Answer from the drawing. Dimensions are ordinates in mm from the lowest x, y and z of the part. A direction names the side the tool comes from. Round coordinates to 2 decimals unless told otherwise and drop trailing zeros. Order: outer loops, then holes, each group sorted by start corner. A loop starts at its lowest first (then second) coordinate and runs counter-clockwise, first axis right, second up. Notation, with made-up numbers: (51, -30.75) -> (91, -30.75) arc R25 cw to (91, -17.75) -> close; hole circle Ø10 at (11.5, -15). An arc over 180 degrees is marked (long way). Use a Markdown table: item, result. Add a question column.
1. Given pin 1 (1 mm diameter, centred on x = 50, z = 59.5, fed in from +Y); pin 2 (2 mm diameter, centred on x = 43.5, y = 46.5, fed in from -Z); pin 3 (14 mm diameter, centred on x = 33, y = 80, fed in from +Z), each flat-ended and moving along its own axis, determine where each tip first touches the part or whether it passes through.
2. Section B-B, the plane x = 34 is taken. Give the vertices of the cut face in (y, z), then the cut area to 3 significant figures.
3. Section A-A, the plane z = 30.5 is taken. Give the vertices of the cut face in (x, y) (1 decimal).
4. Section D-D, the plane z = 22.5 is taken. Give the vertices of the cut face in (x, y), then the cut area to 3 significant figures.
5. Section C-C, the plane y = 81 is taken. Give the vertices of the cut face in (x, z) (1 decimal).
6. For the marked faces 1, 2 and 3, determine the directions among +Z, -Z, +X, -X, +Y, -Y from which every point of the face is accessible in a straight line to the end or side of a thin tool.
7. Consider L1, parallel to Y at x = 23, z = 25.5; L2, parallel to X at y = 96.5, z = 34.5 (1 decimal); L3, parallel to X at y = 41.5, z = 61.5. Determine where each line is inside the solid, lowest interval first. Write a range as [from, to].
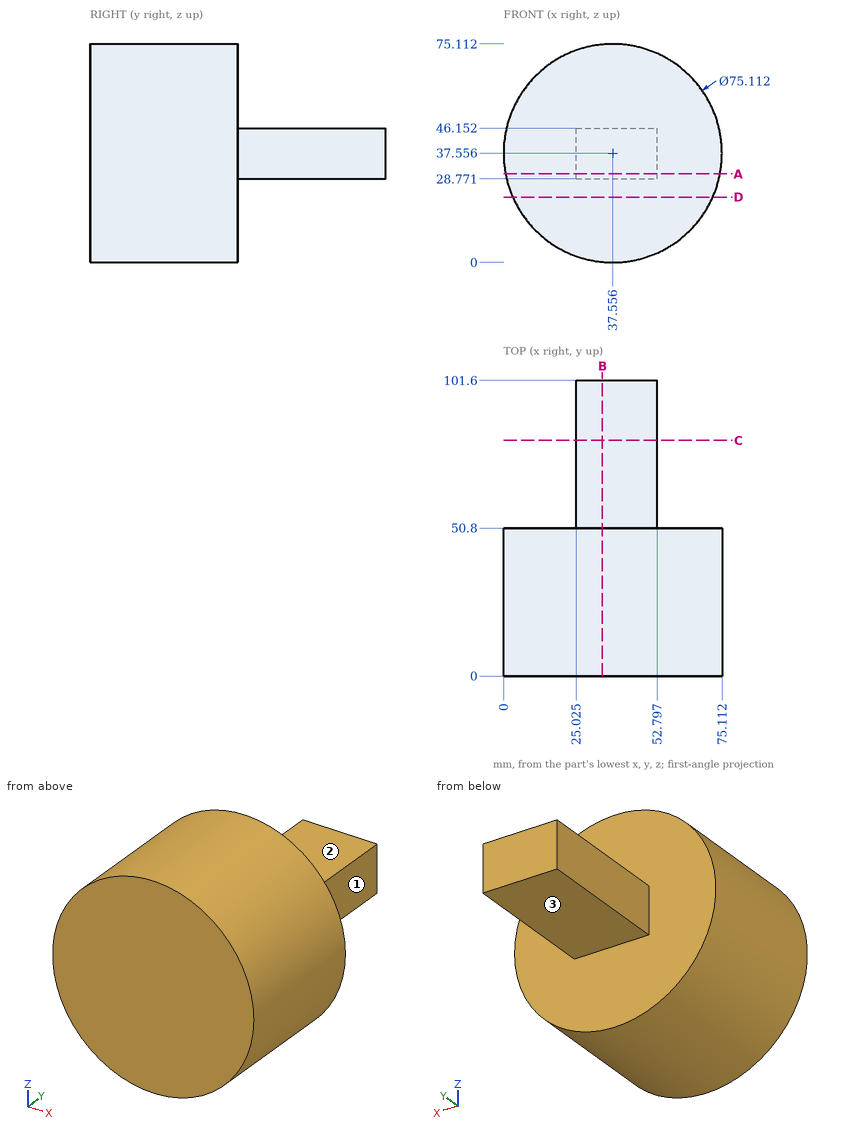
Verdict:
| question | item | result |
|---|---|---|
| 1 | pin 1 | stops at y = 50.8 |
| 1 | pin 2 | stops at z = 0.33 |
| 1 | pin 3 | stops at z = 46.15 |
| 2 | outline | (0, 0.17) -> (50.8, 0.17) -> (50.8, 28.77) -> (101.6, 28.77) -> (101.6, 46.15) -> (50.8, 46.15) -> (50.8, 74.94) -> (0, 74.94) -> close |
| 2 | area | 4,680 mm2 |
| 3 | outline | (0.7, 0) -> (74.4, 0) -> (74.4, 50.8) -> (52.8, 50.8) -> (52.8, 101.6) -> (25, 101.6) -> (25, 50.8) -> (0.7, 50.8) -> close |
| 4 | outline | (3.15, 0) -> (71.96, 0) -> (71.96, 50.8) -> (3.15, 50.8) -> close |
| 4 | area | 3,500 mm2 |
| 5 | outline | (25, 28.8) -> (52.8, 28.8) -> (52.8, 46.2) -> (25, 46.2) -> close |
| 6 | face 1 | +Z, -Z, +X, +Y |
| 6 | face 2 | +Z, +X, -X, +Y |
| 6 | face 3 | -Z, +X, -X, +Y |
| 7 | L1 | y = [0, 50.8] |
| 7 | L2 | x = [25, 52.8] |
| 7 | L3 | x = [8.62, 66.49] |
